Model file for the job. Use its own axes, mm. Face numbers are marked on the shaded views. A direction names the side the tool comes from. Round coordinates to 2 decimals unless told otherwise and drop trailing zeros. Loops run counter-clockwise (first coordinate to the right, second up) from the corner with the lowest first, then second, coordinate; pieces in that order, holes last. Notation, with made-up numbers: M 81.5,49 L 93.5,49 A24 cw 93.5,59 Z; hole C -2.75,59 d10. An arc over 180 degrees is marked long. Use a Markdown table: item, result. Add a question column.
Q1. Cut at B-B (x = -31.5). Give the cut face in (y, z), plus the area to 3 significant figures.
Q2. Pin check, flat tip, straight feed: pin 1 (1 mm diameter, centred on x = 8.5, y = 37, fed in from +Z). Stop position of the tip, or through.
Q3. Cut at C-C (y = -52.5). Give the cut face in (x, z), plus the area to 3 significant figures.
Q4. Cut at A-A (z = 2). Give the cut face in (x, y), plus the area to 3 significant figures.
Q5. Probe line 1 (Y direction, x = 19, z = 6); line 2 (X direction, y = 55, z = 4); line 3 (Z direction, x = 7.5, y = -18.5). List the from-to ranges inside material, lowest first. Write a range as from..to.
Q6. Tool access for the marked faces 1 and 2: list every direction of +Z, -Z, +X, -X, +Y, -Y with a clear straight run to the whole face (end or side of a thin tool).
Q7. Mould opens along Y. For the marked faces 3, 4 and 5 say: +Y half, -Y half, draft (parallel to the pull), parting line (faces both ways), or undercut.
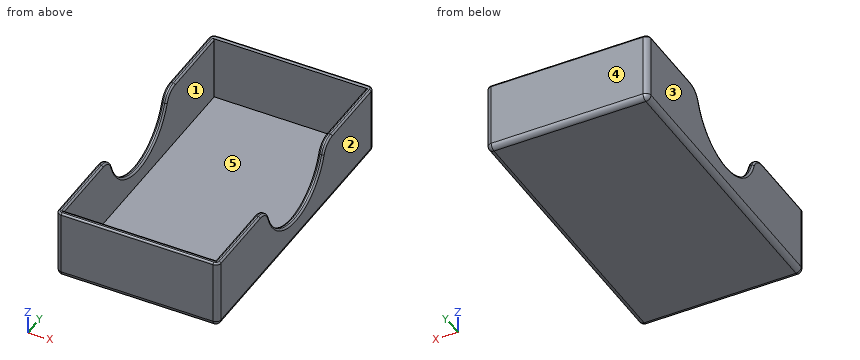
from build123d import *

# Parameters (mm, degrees)
SKETCH014_W          = 70.4
SKETCH014_H          = 130.4
PAD004_DEPTH         = 30
THICKNESS_T          = 2.4
POCKET005_DEPTH      = 37.601
POCKET005_DEPTH_BACK = 37.601
FILLET006_R          = 0.8


with BuildPart() as part:
    # Sketch014 → Pad004 (new body)
    with BuildSketch(Plane.XY):
        Rectangle(SKETCH014_W, SKETCH014_H)
    extrude(amount=PAD004_DEPTH)

    # Thickness
    thickness_openings = [part.faces().sort_by_distance(p)[0] for p in [
        (0, 0, 30),
    ]]
    offset(amount=THICKNESS_T, openings=thickness_openings)

    # Sketch015 → Pocket005 (cut, two sides)
    with BuildSketch(Plane.YZ) as pocket005_sk:
        with BuildLine():
            ThreePointArc((-23.675182, 24.569697), (0, 7.6), (23.675182, 24.569697))
            ThreePointArc((31.25124, 30), (26.590638, 28.502214), (23.675182, 24.569697))
            Line((-31.25124, 30), (31.25124, 30))
            ThreePointArc((-23.675182, 24.569697), (-26.590638, 28.502214), (-31.25124, 30))
        make_face()
    extrude(amount=-POCKET005_DEPTH, mode=Mode.SUBTRACT)
    extrude(pocket005_sk.sketch, amount=POCKET005_DEPTH_BACK, mode=Mode.SUBTRACT)

    # Fillet006
    fillet006_edges = [part.edges().sort_by_distance(p)[0] for p in [
        (0, -65.2, 30),
        (35.2, -48.22562, 30),
        (36.4, -31.25124, 30),
        (37.6, -48.22562, 30),
        (36.897056, -66.897056, 30),
        (0, -67.6, 30),
        (-36.897056, -66.897056, 30),
        (-37.6, -48.22562, 30),
        (-36.4, -31.25124, 30),
        (-35.2, -48.22562, 30),
    ]]
    fillet(fillet006_edges, radius=FILLET006_R)


solid = part.part
Checked values:
| question | item | result |
|---|---|---|
| 1 | outline | M -67.6,0 A2.4 ccw -65.2,-2.4 L 65.2,-2.4 A2.4 ccw 67.6,0 L 67.6,29.2 A0.8 ccw 66.8,30 L 65.2,30 L 65.2,0 L -65.2,0 L -65.2,29.2 A0.8 ccw -66,30 L -66.8,30 A0.8 ccw -67.6,29.2 Z |
| 1 | area | 466 mm^2 |
| 2 | pin 1 | stops at z = 0 |
| 3 | outline | M -37.6,0 A2.4 ccw -35.2,-2.4 L 35.2,-2.4 A2.4 ccw 37.6,0 L 37.6,29.2 A0.8 ccw 36.8,30 L 36,30 A0.8 ccw 35.2,29.2 L 35.2,0 L -35.2,0 L -35.2,29.2 A0.8 ccw -36,30 L -36.8,30 A0.8 ccw -37.6,29.2 Z |
| 3 | area | 321 mm^2 |
| 4 | outline | M -37.6,-65.2 A2.4 ccw -35.2,-67.6 L 35.2,-67.6 A2.4 ccw 37.6,-65.2 L 37.6,65.2 A2.4 ccw 35.2,67.6 L -35.2,67.6 A2.4 ccw -37.6,65.2 Z; hole M -35.2,-65.2 L 35.2,-65.2 L 35.2,65.2 L -35.2,65.2 Z |
| 4 | area | 982 mm^2 |
| 5 | line 1 | y = -67.6..-65.2, 65.2..67.6 |
| 5 | line 2 | x = -37.6..-35.2, 35.2..37.6 |
| 5 | line 3 | z = -2.4..0 |
| 6 | face 1 | +Z |
| 6 | face 2 | +Z, -Z, +X, +Y, -Y |
| 7 | face 3 | draft |
| 7 | face 4 | +Y half |
| 7 | face 5 | undercut |
